Can you work these out from the model? Positions are in its coordinate system, mm. A direction names the side the tool comes from. Round coordinates to 2 decimals unless told otherwise and drop trailing zeros. Write each loop counter-clockwise with the first axis right and the second up, starting at its lowest first coordinate (ties: lowest second). Pieces come first, ordered by that corner, then holes. Notation, with made-up numbers: (5, 32) - (38, 32) arc R21 cw to (38, 53) - close; hole circle Ø5 at (23.25, -36.75). An arc over 180 degrees is marked (long way). One line per item, written item: value. Start each with the question number.
(1) I want a section at C-C on y = -32.5. List the corners of the cut face in (x, z) for me.
(2) On a 3-axis mill with a long thin cutter (end or side, diameter ignored), from which of +Z, -Z, +X, -X, +Y, -Y can I reach the whole of each face in a straight line? I mean faces 1 (the face through (0, 2.032, 4)), 2 (the face through (-4, 12.192, 5)), 3 (the face through (-4, 0, 4)). Say none if no direction works.
(3) I want a section at D-D on y = 3. List the corners of the cut face in (x, z) for me.
(4) I'm going to push flat-ended pins straight in: pin 1 Ø1 at (x, y) = (-4.5, 2) entering from +Z; pin 2 Ø1.5 at (x, z) = (1, 1) entering from +Y; pin 3 Ø3 at (x, y) = (-5, -28) entering from +Z; pin 4 Ø10 at (x, y) = (6, 1.5) entering from -Z. Where does each tip first touch, or does it pass through?
(5) Thinking about a two-plate mould opening in Z: for faces 4 (the face through (-2.321, -36.322, 0.74)), 5 (the face through (1.707, 7.041, 7.687)), 6 (the face through (2.325, -17.907, -1.783)), which applies, +Z half, -Z half, draft (parallel to the pull), parting line (faces both ways), or undercut?
(6) I want a section at A-A on x = 0. List the corners of the cut face in (y, z) for me, plus the area to 3 significant figures.
(7) If I drill on L1, parallel to X at y = 0.8, z = 0; L2, parallel to Y at x = -4.5, z = 6.5, over which ranges is the centre line in solid material (lowest first)? Write a range as from..to.
(8) I want a section at B-B on z = 0. List the corners of the cut face in (x, y) for me.
Autodesk Fusion 360 part; units mm, degrees
sketch "Sketch1" plane through (0, 0, 0) normal (0, 0, 1) x (1, 0, 0)
  line L0 (0, 0) -> (0, -36.322)
  line L1 (0, -36.322) -> (-2.286, -36.322)
  line L2 (-3.556, 0) -> (-2.286, -36.322)
  line L3 (-3.556, 0) -> (-3.556, 2.032)
  line L4 (0, 33.02) -> (0, -60.96) construction
  line L5 (-3.556, 2.032) -> (-5.7945, 2.032)
  line L6 (-6.096, 12.192) -> (0, 12.192)
  line L7 (0, 12.192) -> (0, 0)
  line L8 (-6.096, 12.192) -> (-5.7945, 2.032)
  dimension "d1" = 3.556
  dimension "d2" = 36.322
  dimension "d3" = 2.286
  dimension "d4" = 2.032
  dimension "d8" = 6.096
  dimension "d19" = 88.3
sketch "Sketch2" plane through (0, 0, 0) normal (0, 0, 1) x (1, 0, 0)
  line L0 (-6.096, 12.192) -> (0, 12.192) construction
  line L1 (-6.096, 2.032) -> (-6.096, 12.192) construction
  line L2 (-3.556, 2.032) -> (-5.7945, 2.032) construction
  line L3 (-3.556, 0) -> (-3.556, 2.032) construction
  line L4 (-3.556, 0) -> (-2.286, -36.322) construction
  line L5 (0, -36.322) -> (-2.286, -36.322) construction
  line L6 (-7.874, 12.192) -> (-7.874, 2.032)
  line L7 (-9.3224, 0) -> (-9.3224, 2.032)
  line L8 (-7.874, 2.032) -> (-9.3224, 2.032)
  line L9 (-9.3224, 0) -> (-5.081, 0)
  line L10 (-7.874, 12.192) -> (0, 12.192)
  line L11 (0, 12.192) -> (0, -36.322)
  line L12 (0, -36.322) -> (-3.556, -36.322)
  line L13 (-3.556, -36.322) -> (-5.081, 0)
  dimension "d9" = 1.778
  dimension "d10" = 10.16
  dimension "d12" = 2.032
  dimension "d22" = 3.556
revolve "Revolve1" add sketch "Sketch2" angle 360 about axis through (0, 12.192, 0) along (0, -1, 0)
revolve "Revolve2" cut sketch "Sketch1" angle 360 about axis through (0, 12.192, 0) along (0, -1, 0)
fillet "Fillet1" radius 0.889 2 edges at (-8.6915, 2.032, 3.3711) (-8.6915, 0, 3.3711)
Established:
1. outline: circle Ø7.43 at (0, 0); hole circle Ø4.84 at (0, 0)
2. face 1: +Y
2. face 2: +Z, -Z, +X, -X, +Y
2. face 3: -Y
3. outline: circle Ø15.75 at (0, 0); hole circle Ø11.65 at (0, 0)
4. pin 1: z = 8.18
4. pin 2: through
4. pin 3: z = 1.74
4. pin 4: z = -9.27
5. face 4: draft
5. face 5: parting line
5. face 6: undercut
6. outline: (-36.32, -3.56) - (0, -5.08) - (0, -8.43) arc R0.89 ccw to (0.89, -9.32) - (1.14, -9.32) arc R0.89 ccw to (2.03, -8.43) - (2.03, -7.87) - (12.19, -7.87) - (12.19, -6.1) - (2.03, -5.79) - (2.03, -3.56) - (0, -3.56) - (-36.32, -2.29) - close; (-36.32, 2.29) - (0, 3.56) - (2.03, 3.56) - (2.03, 5.79) - (12.19, 6.1) - (12.19, 7.87) - (2.03, 7.87) - (2.03, 8.43) arc R0.89 ccw to (1.14, 9.32) - (0.89, 9.32) arc R0.89 ccw to (0, 8.43) - (0, 5.08) - (-36.32, 3.56) - close
6. area: 163 mm2
7. L1: -9.32..-3.56, 3.56..9.32
7. L2: 0..2.03
8. outline: (-9.32, 0.89) arc R0.89 ccw to (-8.43, 0) - (-5.08, 0) - (-3.56, -36.32) - (-2.29, -36.32) - (-3.56, 0) - (-3.56, 2.03) - (-5.79, 2.03) - (-6.1, 12.19) - (-7.87, 12.19) - (-7.87, 2.03) - (-8.43, 2.03) arc R0.89 ccw to (-9.32, 1.14) - close; (2.29, -36.32) - (3.56, -36.32) - (5.08, 0) - (8.43, 0) arc R0.89 ccw to (9.32, 0.89) - (9.32, 1.14) arc R0.89 ccw to (8.43, 2.03) - (7.87, 2.03) - (7.87, 12.19) - (6.1, 12.19) - (5.79, 2.03) - (3.56, 2.03) - (3.56, 0) - close
